Design review of the part built by this model. Coordinates are the model's own, in mm. A direction names the side the tool comes from. Coordinates: 2 decimals unless noted, no trailing zeros. Loops run counter-clockwise (first coordinate to the right, second up) from the corner with the lowest first, then second, coordinate; pieces in that order, holes last. Notation, with made-up numbers: (-15.75, 57) - (12.25, 57) arc R4 cw to (12.25, 62) - close; hole circle Ø5 at (53, 21.5). An arc over 180 degrees is marked (long way). Return JSON: item names as keys, results as strings. Group by question number.
from build123d import *

# Parameters (mm, degrees)
SKETCH1_W                  = 51
SKETCH1_H                  = 28.56
TOTALHEIGHT_DEPTH          = 15
SKETCH1_3_W                = 51
SKETCH1_3_H                = 28.56
FLOORHEIGHT_DEPTH          = 2.5
HOLESFORBEARINGMOUNT_REACH = 139.241
SKETCH2_R                  = 1.55
SKETCH2_R_2                = 3.5
CUT_EXTRUDE2_REACH         = 131.019


with BuildPart() as part:
    # Sketch1 → TotalHeight (new body)
    with BuildSketch(Plane(origin=(0, 0, 0), x_dir=(1, 0, 0), z_dir=(0, 1, 0))):
        Polygon((32, 32), (32, 0), (89, 0), (89, 32), (121, 32), (121, 47.5), (121, 63), (89, 63), (89, 95), (32, 95), (32, 63), (0, 63), (0, 58), (5, 58), (116, 58), (116, 37), (5, 37), (0, 37), (0, 32), align=None)
        with Locations((60.5, 17.72)):
            Rectangle(SKETCH1_W, SKETCH1_H, mode=Mode.SUBTRACT)
        with Locations((60.5, 77.28)):
            Rectangle(SKETCH1_W, SKETCH1_H, mode=Mode.SUBTRACT)
    extrude(amount=TOTALHEIGHT_DEPTH)

    # Sketch1<3> → FloorHeight (add)
    # profile 1 of 2: a face of its own
    with BuildSketch(Plane(origin=(0, 0, 0), x_dir=(1, 0, 0), z_dir=(0, 1, 0))):
        with Locations((60.5, 77.28)):
            Rectangle(SKETCH1_3_W, SKETCH1_3_H)
        with BuildLine():
            ThreePointArc((78, 79.17), (83.25, 84.42), (78, 89.67))
            Line((78, 89.67), (43, 89.67))
            ThreePointArc((43, 89.67), (37.75, 84.42), (43, 79.17))
            Line((43, 79.17), (78, 79.17))
        make_face(mode=Mode.SUBTRACT)
        with BuildLine():
            Line((43, 75.39), (78, 75.39))
            ThreePointArc((78, 75.39), (83.25, 70.14), (78, 64.89))
            Line((78, 64.89), (43, 64.89))
            ThreePointArc((43, 64.89), (37.75, 70.14), (43, 75.39))
        make_face(mode=Mode.SUBTRACT)
    # profile 2 of 2: a face of its own
    with BuildSketch(Plane(origin=(0, 0, 0), x_dir=(1, 0, 0), z_dir=(0, 1, 0))):
        with Locations((60.5, 17.72)):
            Rectangle(SKETCH1_3_W, SKETCH1_3_H)
        with BuildLine():
            ThreePointArc((78, 19.61), (83.25, 24.86), (78, 30.11))
            Line((78, 30.11), (43, 30.11))
            ThreePointArc((43, 30.11), (37.75, 24.86), (43, 19.61))
            Line((43, 19.61), (78, 19.61))
        make_face(mode=Mode.SUBTRACT)
        with BuildLine():
            Line((43, 15.83), (78, 15.83))
            ThreePointArc((78, 15.83), (83.25, 10.58), (78, 5.33))
            Line((78, 5.33), (43, 5.33))
            ThreePointArc((43, 5.33), (37.75, 10.58), (43, 15.83))
        make_face(mode=Mode.SUBTRACT)
    extrude(amount=FLOORHEIGHT_DEPTH)

    # HolesForBearingMount: up to this face of the body (flat: up to its plane)
    holesforbearingmount_end = Plane(part.part.faces().sort_by_distance((16, 7.5, -63))[0])
    # Sketch2 → HolesForBearingMount (cut, up to the picked face)
    with BuildSketch(Plane.XY.offset(-32), mode=Mode.PRIVATE) as holesforbearingmount_sk1:
        with Locations((2.45, 6)):
            Circle(SKETCH2_R)
    holesforbearingmount_tool1 = split(extrude(holesforbearingmount_sk1.sketch, amount=-HOLESFORBEARINGMOUNT_REACH, mode=Mode.PRIVATE), bisect_by=holesforbearingmount_end, keep=Keep.BOTH, mode=Mode.PRIVATE)
    # Sketch2 → HolesForBearingMount (cut, up to the picked face)
    with BuildSketch(Plane.XY.offset(-32), mode=Mode.PRIVATE) as holesforbearingmount_sk2:
        with Locations((13.7, 6)):
            Circle(SKETCH2_R_2)
    holesforbearingmount_tool2 = split(extrude(holesforbearingmount_sk2.sketch, amount=-HOLESFORBEARINGMOUNT_REACH, mode=Mode.PRIVATE), bisect_by=holesforbearingmount_end, keep=Keep.BOTH, mode=Mode.PRIVATE)
    # Sketch2 → HolesForBearingMount (cut, up to the picked face)
    with BuildSketch(Plane.XY.offset(-32), mode=Mode.PRIVATE) as holesforbearingmount_sk3:
        with BuildLine():
            Line((24.95, 4.45), (27.95, 4.45))
            ThreePointArc((27.95, 4.45), (29.5, 6), (27.95, 7.55))
            Line((27.95, 7.55), (24.95, 7.55))
            ThreePointArc((24.95, 7.55), (23.4, 6), (24.95, 4.45))
        make_face()
    holesforbearingmount_tool3 = split(extrude(holesforbearingmount_sk3.sketch, amount=-HOLESFORBEARINGMOUNT_REACH, mode=Mode.PRIVATE), bisect_by=holesforbearingmount_end, keep=Keep.BOTH, mode=Mode.PRIVATE)
    # Sketch2 → HolesForBearingMount (cut, up to the picked face)
    with BuildSketch(Plane.XY.offset(-32), mode=Mode.PRIVATE) as holesforbearingmount_sk4:
        with BuildLine():
            ThreePointArc((93.05, 4.45), (91.5, 6), (93.05, 7.55))
            Line((93.05, 7.55), (96.05, 7.55))
            ThreePointArc((96.05, 7.55), (97.6, 6), (96.05, 4.45))
            Line((96.05, 4.45), (93.05, 4.45))
        make_face()
    holesforbearingmount_tool4 = split(extrude(holesforbearingmount_sk4.sketch, amount=-HOLESFORBEARINGMOUNT_REACH, mode=Mode.PRIVATE), bisect_by=holesforbearingmount_end, keep=Keep.BOTH, mode=Mode.PRIVATE)
    # Sketch2 → HolesForBearingMount (cut, up to the picked face)
    with BuildSketch(Plane.XY.offset(-32), mode=Mode.PRIVATE) as holesforbearingmount_sk5:
        with Locations((107.3, 6)):
            Circle(SKETCH2_R_2)
    holesforbearingmount_tool5 = split(extrude(holesforbearingmount_sk5.sketch, amount=-HOLESFORBEARINGMOUNT_REACH, mode=Mode.PRIVATE), bisect_by=holesforbearingmount_end, keep=Keep.BOTH, mode=Mode.PRIVATE)
    add(holesforbearingmount_tool1.solids().sort_by(Axis((2.45, 6, -32), (0, 0, -1)))[0], mode=Mode.SUBTRACT)
    add(holesforbearingmount_tool2.solids().sort_by(Axis((13.7, 6, -32), (0, 0, -1)))[0], mode=Mode.SUBTRACT)
    add(holesforbearingmount_tool3.solids().sort_by(Axis((26.45, 6, -32), (0, 0, -1)))[0], mode=Mode.SUBTRACT)
    add(holesforbearingmount_tool4.solids().sort_by(Axis((94.55, 6, -32), (0, 0, -1)))[0], mode=Mode.SUBTRACT)
    add(holesforbearingmount_tool5.solids().sort_by(Axis((107.3, 6, -32), (0, 0, -1)))[0], mode=Mode.SUBTRACT)

    # Cut-Extrude2: up to this face of the body (flat: up to its plane)
    cut_extrude2_end = Plane(part.part.faces().sort_by_distance((35, 8.75, -17.72))[0])
    # Sketch3 → Cut-Extrude2 (cut, up to the picked face)
    with BuildSketch(Plane.ZY.offset(-86), mode=Mode.PRIVATE) as cut_extrude2_sk1:
        with BuildLine():
            ThreePointArc((-77.36, 8), (-87.503934876, 14.414394786), (-88.949988864, 2.5))
            Line((-88.949988864, 2.5), (-79.970011136, 2.5))
            ThreePointArc((-79.970011136, 2.5), (-78.045605214, 4.956065124), (-77.36, 8))
        make_face()
    cut_extrude2_tool1 = split(extrude(cut_extrude2_sk1.sketch, amount=CUT_EXTRUDE2_REACH, mode=Mode.PRIVATE), bisect_by=cut_extrude2_end, keep=Keep.BOTH, mode=Mode.PRIVATE)
    # Sketch3 → Cut-Extrude2 (cut, up to the picked face)
    with BuildSketch(Plane.ZY.offset(-86), mode=Mode.PRIVATE) as cut_extrude2_sk2:
        with BuildLine():
            Line((-79.970011136, 2.5), (-88.949988864, 2.5))
            ThreePointArc((-88.949988864, 2.5), (-84.46, 0.9), (-79.970011136, 2.5))
        make_face()
    cut_extrude2_tool2 = split(extrude(cut_extrude2_sk2.sketch, amount=CUT_EXTRUDE2_REACH, mode=Mode.PRIVATE), bisect_by=cut_extrude2_end, keep=Keep.BOTH, mode=Mode.PRIVATE)
    # Sketch3 → Cut-Extrude2 (cut, up to the picked face)
    with BuildSketch(Plane.ZY.offset(-86), mode=Mode.PRIVATE) as cut_extrude2_sk3:
        with BuildLine():
            ThreePointArc((-63, 8), (-73.143934876, 14.414394786), (-74.589988864, 2.5))
            Line((-74.589988864, 2.5), (-65.610011136, 2.5))
            ThreePointArc((-65.610011136, 2.5), (-63.685605214, 4.956065124), (-63, 8))
        make_face()
    cut_extrude2_tool3 = split(extrude(cut_extrude2_sk3.sketch, amount=CUT_EXTRUDE2_REACH, mode=Mode.PRIVATE), bisect_by=cut_extrude2_end, keep=Keep.BOTH, mode=Mode.PRIVATE)
    # Sketch3 → Cut-Extrude2 (cut, up to the picked face)
    with BuildSketch(Plane.ZY.offset(-86), mode=Mode.PRIVATE) as cut_extrude2_sk4:
        with BuildLine():
            Line((-65.610011136, 2.5), (-74.589988864, 2.5))
            ThreePointArc((-74.589988864, 2.5), (-70.1, 0.9), (-65.610011136, 2.5))
        make_face()
    cut_extrude2_tool4 = split(extrude(cut_extrude2_sk4.sketch, amount=CUT_EXTRUDE2_REACH, mode=Mode.PRIVATE), bisect_by=cut_extrude2_end, keep=Keep.BOTH, mode=Mode.PRIVATE)
    # Sketch3 → Cut-Extrude2 (cut, up to the picked face)
    with BuildSketch(Plane.ZY.offset(-86), mode=Mode.PRIVATE) as cut_extrude2_sk5:
        with BuildLine():
            ThreePointArc((-17.8, 8), (-27.943934876, 14.414394786), (-29.389988864, 2.5))
            Line((-29.389988864, 2.5), (-20.410011136, 2.5))
            ThreePointArc((-20.410011136, 2.5), (-18.485605214, 4.956065124), (-17.8, 8))
        make_face()
    cut_extrude2_tool5 = split(extrude(cut_extrude2_sk5.sketch, amount=CUT_EXTRUDE2_REACH, mode=Mode.PRIVATE), bisect_by=cut_extrude2_end, keep=Keep.BOTH, mode=Mode.PRIVATE)
    # Sketch3 → Cut-Extrude2 (cut, up to the picked face)
    with BuildSketch(Plane.ZY.offset(-86), mode=Mode.PRIVATE) as cut_extrude2_sk6:
        with BuildLine():
            Line((-20.410011136, 2.5), (-29.389988864, 2.5))
            ThreePointArc((-29.389988864, 2.5), (-24.9, 0.9), (-20.410011136, 2.5))
        make_face()
    cut_extrude2_tool6 = split(extrude(cut_extrude2_sk6.sketch, amount=CUT_EXTRUDE2_REACH, mode=Mode.PRIVATE), bisect_by=cut_extrude2_end, keep=Keep.BOTH, mode=Mode.PRIVATE)
    # Sketch3 → Cut-Extrude2 (cut, up to the picked face)
    with BuildSketch(Plane.ZY.offset(-86), mode=Mode.PRIVATE) as cut_extrude2_sk7:
        with BuildLine():
            ThreePointArc((-3.44, 8), (-13.583934876, 14.414394786), (-15.029988864, 2.5))
            Line((-15.029988864, 2.5), (-6.050011136, 2.5))
            ThreePointArc((-6.050011136, 2.5), (-4.125605214, 4.956065124), (-3.44, 8))
        make_face()
    cut_extrude2_tool7 = split(extrude(cut_extrude2_sk7.sketch, amount=CUT_EXTRUDE2_REACH, mode=Mode.PRIVATE), bisect_by=cut_extrude2_end, keep=Keep.BOTH, mode=Mode.PRIVATE)
    # Sketch3 → Cut-Extrude2 (cut, up to the picked face)
    with BuildSketch(Plane.ZY.offset(-86), mode=Mode.PRIVATE) as cut_extrude2_sk8:
        with BuildLine():
            Line((-6.050011136, 2.5), (-15.029988864, 2.5))
            ThreePointArc((-15.029988864, 2.5), (-10.54, 0.9), (-6.050011136, 2.5))
        make_face()
    cut_extrude2_tool8 = split(extrude(cut_extrude2_sk8.sketch, amount=CUT_EXTRUDE2_REACH, mode=Mode.PRIVATE), bisect_by=cut_extrude2_end, keep=Keep.BOTH, mode=Mode.PRIVATE)
    add(cut_extrude2_tool1.solids().sort_by(Axis((86, 8.40623, -84.46), (-1, 0, 0)))[0], mode=Mode.SUBTRACT)
    add(cut_extrude2_tool2.solids().sort_by(Axis((86, 1.853386, -84.46), (-1, 0, 0)))[0], mode=Mode.SUBTRACT)
    add(cut_extrude2_tool3.solids().sort_by(Axis((86, 8.40623, -70.1), (-1, 0, 0)))[0], mode=Mode.SUBTRACT)
    add(cut_extrude2_tool4.solids().sort_by(Axis((86, 1.853386, -70.1), (-1, 0, 0)))[0], mode=Mode.SUBTRACT)
    add(cut_extrude2_tool5.solids().sort_by(Axis((86, 8.40623, -24.9), (-1, 0, 0)))[0], mode=Mode.SUBTRACT)
    add(cut_extrude2_tool6.solids().sort_by(Axis((86, 1.853386, -24.9), (-1, 0, 0)))[0], mode=Mode.SUBTRACT)
    add(cut_extrude2_tool7.solids().sort_by(Axis((86, 8.40623, -10.54), (-1, 0, 0)))[0], mode=Mode.SUBTRACT)
    add(cut_extrude2_tool8.solids().sort_by(Axis((86, 1.853386, -10.54), (-1, 0, 0)))[0], mode=Mode.SUBTRACT)


solid = part.part
Item 1: To check wall thickness, follow line 1 (Z direction, x = 50, y = 8.25); line 2 (Z direction, x = 52, y = 0.75); line 3 (Y direction, x = 107.3, z = -35.1). State the ranges of each line that lie inside material, in increasing order. Write a range as from..to.
Item 2: Add section D-D (z = -70.14). State the section outline as (x, y) points.
Item 3: Add section B-B (x = 102). State the section outline as (y, z) points.
Item 4: For P1, Ø5, axis at x = 68.5, y = 3.5, coming from the +Z side; P2, Ø2, axis at x = 66, z = -65, coming from the +Y side; P3, Ø3, axis at y = 5, z = -22.5, coming from the -X side; P4, Ø3.5, axis at x = 2.45, y = 6, coming from the +Z side, all flat-tipped, find the tip position at first contact; note any pin that passes through.
Item 5: Add section C-C (y = 12). State the section outline as (x, z) points, then the cut area to 3 significant figures.
Item 6: For faces 1 (the face through (105, 9, -32)), 2 (the face through (116, 7, -48)), 3 (the face through (35, 8, -77)), list the 3-axis set-ups (+Z, -Z, +X, -X, +Y, -Y) from which the entire face can be reached by the end or side of a thin tool; tool diameter is ignored.
Item 7: Add section A-A (x = 2.45). State the section outline as (y, z) points.
Item 8: Draft analysis for pull direction Y (two halves, no side actions). For faces 4 (the face through (84, 0.9, -84.5)), 5 (the face through (29.5, 6, -60.5)), 6 (the face through (89, 7, -16)), state which applies: pulls with the +Y half, pulls with the -Y half, needs draft (parallel to the pull), parting line crosses it, or undercut.
Answers below:
{
 "1": {"line 1": "z = -95..-91.56, -63..-58, -37..-32, -3.44..0", "line 2": "z = -95..-89.67, -79.17..-75.39, -64.89..-58, -37..-30.11, -19.61..-15.83, -5.33..0", "line 3": "y = 0..2.5, 9.5..15"},
 "2": {"outline": "(32, 0) - (37.75, 0) - (37.75, 0.9) - (35, 0.9) - (35, 15) - (32, 15) - close; (83.25, 0) - (89, 0) - (89, 15) - (86, 15) - (86, 0.9) - (83.25, 0.9) - close"},
 "3": {"outline": "(0, -63) - (15, -63) - (15, -58) - (0, -58) - close; (0, -37) - (15, -37) - (15, -32) - (0, -32) - close"},
 "4": {"P1": "stops at z = 0", "P2": "stops at y = 2.5", "P3": "stops at x = 32", "P4": "stops at z = -32"},
 "5": {"outline": "(0, -63) - (32, -63) - (32, -95) - (89, -95) - (89, -63) - (121, -63) - (121, -32) - (89, -32) - (89, 0) - (32, 0) - (32, -32) - (0, -32) - (0, -37) - (116, -37) - (116, -58) - (0, -58) - close; hole (35, -91.56) - (86, -91.56) - (86, -63) - (35, -63) - close; hole (35, -32) - (86, -32) - (86, -3.44) - (35, -3.44) - close", "area": "2,050 mm^2"},
 "6": {"face 1": "+Z, +X, +Y, -Y", "face 2": "-X, +Y, -Y", "face 3": "+Y"},
 "7": {"outline": "(0, -63) - (4.45, -63) - (4.45, -58) - (0, -58) - close; (0, -37) - (4.45, -37) - (4.45, -32) - (0, -32) - close; (7.55, -63) - (15, -63) - (15, -58) - (7.55, -58) - close; (7.55, -37) - (15, -37) - (15, -32) - (7.55, -32) - close"},
 "8": {"face 4": "pulls with the +Y half", "face 5": "undercut", "face 6": "needs draft"}
}
